from build123d import *

# Parameters (mm, degrees)
F2_R     = 25
F3_DEPTH = 87.7511


with BuildPart() as f1:
    # F0 (on Front) → F1 (revolve)
    with BuildSketch(Plane.XZ):
        with BuildLine():
            ThreePointArc((245, 0), (129.298665, -61.504004), (0, -82.7501))
            Line((0, -82.7501), (0, -87.7501))
            ThreePointArc((0, -87.7501), (132.476489, -65.175563), (250, 0))
            Line((250, 0), (250, 600))
            Line((250, 600), (352.5, 600))
            Line((352.5, 600), (352.5, 636))
            Line((352.5, 636), (245, 636))
            Line((245, 636), (245, 0))
        make_face()
    revolve(axis=Axis((0, 0, 24.765719), (0, 0, -1)))

    # F2 (on Top) → F3 (cut, through all)
    with BuildSketch(Plane.XY):
        Circle(F2_R)
    extrude(amount=-F3_DEPTH, mode=Mode.SUBTRACT)


solid = f1.part
The listing builds one solid part. Answer for the finished solid, in the listing's coordinates (mm). A direction names the side the tool comes from. Round coordinates to 2 decimals unless told otherwise and drop trailing zeros. Order: outer loops, then holes, each group sorted by start corner. A loop starts at its lowest first (then second) coordinate and runs counter-clockwise, first axis right, second up. Notation, with made-up numbers: (72.5, -35) - (98.5, -35) arc R32 ccw to (98.5, 3) - close; hole circle Ø4 at (29, -31). An arc over 180 degrees is marked (long way). Write item = value, one per line. Start each with the question number.
1) For a pull along X with two mould halves and no side action, classify faces 1 (the cylindrical face through (23.846, 7.509, -84.437)), 2 (the flat face through (-73, -240, 600)), 3 (the cylindrical face through (-249.76, -10.99, 304.2)) as released by +X, released by -X, zero draft, split by the parting line, or undercut.
2) For faces 4 (the cylindrical face through (-76.415, 344.118, 618.252)), 5 (the cylindrical face through (-53.111, 239.174, 313.548)), determine the directions among +Z, -Z, +X, -X, +Y, -Y from which every point of the face is accessible in a straight line to the end or side of a thin tool.
3) Section A-A, the plane z = 256 is taken. Write down the section's boundary in (x, y), plus the area to 3 significant figures.
4) Straight lines are drawn through the part: L1, parallel to X at y = 0, z = 427; L2, parallel to Y at x = 4, z = 119.5; L3, parallel to Y at x = 60, z = 258.5. For each, find the intervals that lie inside material, in ascending order.
5) Given pin 1 (2 mm diameter, centred on y = -172, z = 28, fed in from +X); pin 2 (12 mm diameter, centred on x = -11.5, y = 36, fed in from -Z); pin 3 (12 mm diameter, centred on y = 0.5, z = 527, fed in from -X), each flat-ended and moving along its own axis, determine where each tip first touches the part or whether it passes through.
Results list:
q1.face_1 = undercut
q1.face_2 = zero draft
q1.face_3 = split by the parting line
q2.face_4 = +Z, -Z
q2.face_5 = +Z
q3.outline = circle Ø500 at (0, 0); hole circle Ø490 at (0, 0)
q3.area = 7,780 mm^2
q4.L1 = -250 to -245, 245 to 250
q4.L2 = -249.97 to -244.97, 244.97 to 249.97
q4.L3 = -242.69 to -237.54, 237.54 to 242.69
q5.pin_1 = 182.37
q5.pin_2 = -86.48
q5.pin_3 = -250
